Could you check a few things on this model? Use its own coordinates, in mm. Face numbers are marked on the shaded views. A direction names the side the tool comes from. Coordinates: 2 decimals unless noted, no trailing zeros. Order: outer loops, then holes, each group sorted by start corner. A loop starts at its lowest first (then second) coordinate and runs counter-clockwise, first axis right, second up. Notation, with made-up numbers: (41, 46.25) - (84, 46.25) arc R35 cw to (84, 84.25) - close; hole circle Ø8 at (-9, 21.5). An arc over 180 degrees is marked (long way). Answer as CSV lines item,"result". Start each with the question number.
1. I want a section at A-A, the plane y = 1589.5. List the corners of the cut face in (x, z) for me.
2. Thinking about a two-plate mould opening in X: for the marked faces 5, 6 and 7, which applies, released by +X, released by -X, zero draft, split by the parting line, or undercut?
3. I need wall thicknesses on probe 1 along X at (y, z) = (1580.5, -0.8); probe 2 along Y at (x, z) = (315.75, -2.4); probe 3 along Y at (x, z) = (316.75, -2.35). Which ranges of each line are inside material? Lowest first, please.
4. I want a section at B-B, the plane x = 318.75. List the corners of the cut face in (y, z) for me.
5. I want a section at D-D, the plane y = 1562.5. List the corners of the cut face in (x, z) for me.
6. I want a section at C-C, the plane z = -0.65. List the corners of the cut face in (x, y) for me.
7. For the marked faces 1, 2, 3 and 4, which set-ups out of +Z, -Z, +X, -X, +Y, -Y let a thin tool reach every point of the face, with its end or its side?
8. For pin 1 (0.9 mm diameter, centred on y = 1603.5, z = -1.5, fed in from -X); pin 2 (1.5 mm diameter, centred on x = 316.55, y = 1556.86, fed in from +Z); pin 3 (1 mm diameter, centred on x = 313.5, z = -0.5, fed in from +Y); pin 4 (1.5 mm diameter, centred on y = 1572.5, z = -1, fed in from +X), each with a flat end and sliding along its axis, tell me the tip position at first contact or that it passes through.
from build123d import *

# Parameters (mm, degrees)
ESQUISSE1_R               = 3.5
ESQUISSE1_R_2             = 1.25
T_LE_DE_BASE_PLI_E1_DEPTH = 3


# Sheet-metal steps are written as plain solids
with BuildPart() as part:
    # Esquisse1 → Tôle de base pliée1 (new body)
    with BuildSketch(Plane.XY):
        with BuildLine():
            Line((312.545394727, 1587.348462935), (312.545394727, 1556.858242671))
            ThreePointArc((312.545394727, 1556.858242671), (316.545394727, 1552.858242671), (320.545394727, 1556.858242671))
            Line((320.545394727, 1556.858242671), (320.545394727, 1587.348462935))
            ThreePointArc((320.545394727, 1587.348462935), (322.545394727, 1591.82059889), (320.545394727, 1596.292734845))
            Line((320.545394727, 1596.292734845), (320.545394727, 1605.02468454))
            ThreePointArc((320.545394727, 1605.02468454), (316.545394727, 1609.02468454), (312.545394727, 1605.02468454))
            Line((312.545394727, 1605.02468454), (312.545394727, 1596.292734845))
            ThreePointArc((312.545394727, 1596.292734845), (310.545394727, 1591.82059889), (312.545394727, 1587.348462935))
        make_face()
        with Locations((316.545394727, 1591.82059889)):
            Circle(ESQUISSE1_R, mode=Mode.SUBTRACT)
        with Locations((316.545394727, 1556.858242671)):
            Circle(ESQUISSE1_R_2, mode=Mode.SUBTRACT)
        with BuildLine():
            Line((315.495394727, 1605.57468454), (315.495394727, 1602.17468454))
            ThreePointArc((315.495394727, 1602.17468454), (316.545394727, 1601.12468454), (317.595394727, 1602.17468454))
            Line((317.595394727, 1602.17468454), (317.595394727, 1605.57468454))
            ThreePointArc((317.595394727, 1605.57468454), (316.545394727, 1606.62468454), (315.495394727, 1605.57468454))
        make_face(mode=Mode.SUBTRACT)
        with BuildLine():
            Line((315.495394727, 1581.87059889), (315.495394727, 1577.17059889))
            ThreePointArc((315.495394727, 1577.17059889), (316.545394727, 1576.12059889), (317.595394727, 1577.17059889))
            Line((317.595394727, 1577.17059889), (317.595394727, 1581.87059889))
            ThreePointArc((317.595394727, 1581.87059889), (316.545394727, 1582.92059889), (315.495394727, 1581.87059889))
        make_face(mode=Mode.SUBTRACT)
    extrude(amount=-T_LE_DE_BASE_PLI_E1_DEPTH)


solid = part.part
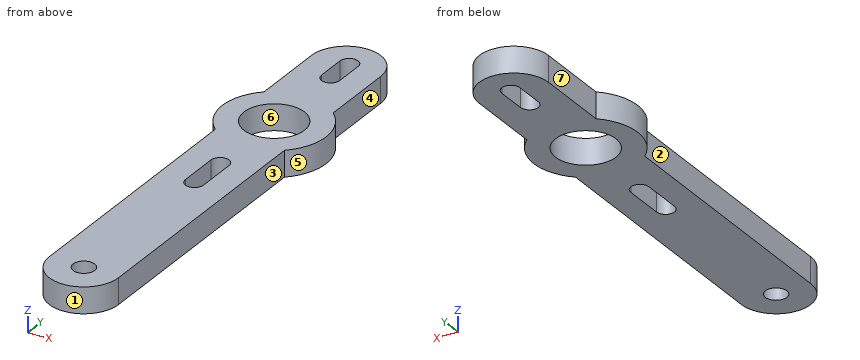
Solved:
1,outline,"(311.01, -3) - (313.93, -3) - (313.93, 0) - (311.01, 0) - close; (319.17, -3) - (322.08, -3) - (322.08, 0) - (319.17, 0) - close"
2,face 5,"released by +X"
2,face 6,"undercut"
2,face 7,"released by -X"
3,probe 1,"x = 312.55 to 315.5, 317.6 to 320.55"
3,probe 2,"y = 1552.94 to 1555.89, 1557.82 to 1576.49, 1582.56 to 1588.41, 1595.23 to 1601.49, 1606.26 to 1608.94"
3,probe 3,"y = 1552.86 to 1555.63, 1558.09 to 1576.14, 1582.9 to 1588.33, 1595.31 to 1601.14, 1606.6 to 1609.02"
4,outline,"(1553.52, -3) - (1589.1, -3) - (1589.1, 0) - (1553.52, 0) - close; (1594.54, -3) - (1608.36, -3) - (1608.36, 0) - (1594.54, 0) - close"
5,outline,"(312.55, -3) - (320.55, -3) - (320.55, 0) - (312.55, 0) - close"
6,outline,"(312.55, 1556.86) arc R4 ccw to (320.55, 1556.86) - (320.55, 1587.35) arc R6 ccw to (320.55, 1596.29) - (320.55, 1605.02) arc R4 ccw to (312.55, 1605.02) - (312.55, 1596.29) arc R6 ccw to (312.55, 1587.35) - close; hole circle Ø7 at (316.55, 1591.82); hole circle Ø2.5 at (316.55, 1556.86); hole (315.5, 1577.17) arc R1.05 ccw to (317.6, 1577.17) - (317.6, 1581.87) arc R1.05 ccw to (315.5, 1581.87) - close; hole (315.5, 1602.17) arc R1.05 ccw to (317.6, 1602.17) - (317.6, 1605.57) arc R1.05 ccw to (315.5, 1605.57) - close"
7,face 1,"+Z, -Z, -Y"
7,face 2,"+Z, -Z, -X, -Y"
7,face 3,"+Z, -Z, +X, -Y"
7,face 4,"+Z, -Z, +X, +Y"
8,pin 1,"stops at x = 312.55"
8,pin 2,"passes through"
8,pin 3,"stops at y = 1608.11"
8,pin 4,"stops at x = 320.55"
